Study the drawing (mm; zero at the part's minimum x, y, z) and answer. A direction names the side the tool comes from. Coordinates: 2 decimals unless noted, no trailing zeros. Write each loop counter-clockwise with the first axis right and the second up, starting at its lowest first coordinate (ties: lowest second). Pieces come first, ordered by that corner, then holes. Notation, with made-up numbers: (-23, 43) -> (17, 43) arc R20 cw to (17, 72) -> close; hole circle Ø1 at (10.25, 11). An arc over 180 degrees is marked (long way). Answer in a Markdown table with one row per item. Add a question column.
Item 1: Section B-B on x = 110.5 is taken. Write down the section's boundary in (y, z).
Item 2: Given pin 1 Ø12 at (x, y) = (30, 64.5) entering from -Z; pin 2 Ø3 at (x, y) = (14, 101.5) entering from +Z, each flat-ended and moving along its own axis, determine where each tip first touches the part or whether it passes through.
Item 3: Which of the six approach directions +Z, -Z, +X, -X, +Y, -Y give full straight-line access (tool end or side, diameter ignored) to the marked faces 1, 2 and 3?
Item 4: Straight lines are drawn through the part: line 1 (Z direction, x = 122.5, y = 21); line 2 (Y direction, x = 22.5, z = 41.5); line 3 (Y direction, x = 21.5, z = 71.5). For each, find the intervals that lie inside material, in ascending order. Write a range as from..to.
Item 5: Section A-A on y = 35.5 is taken. Write down the section's boundary in (x, z).
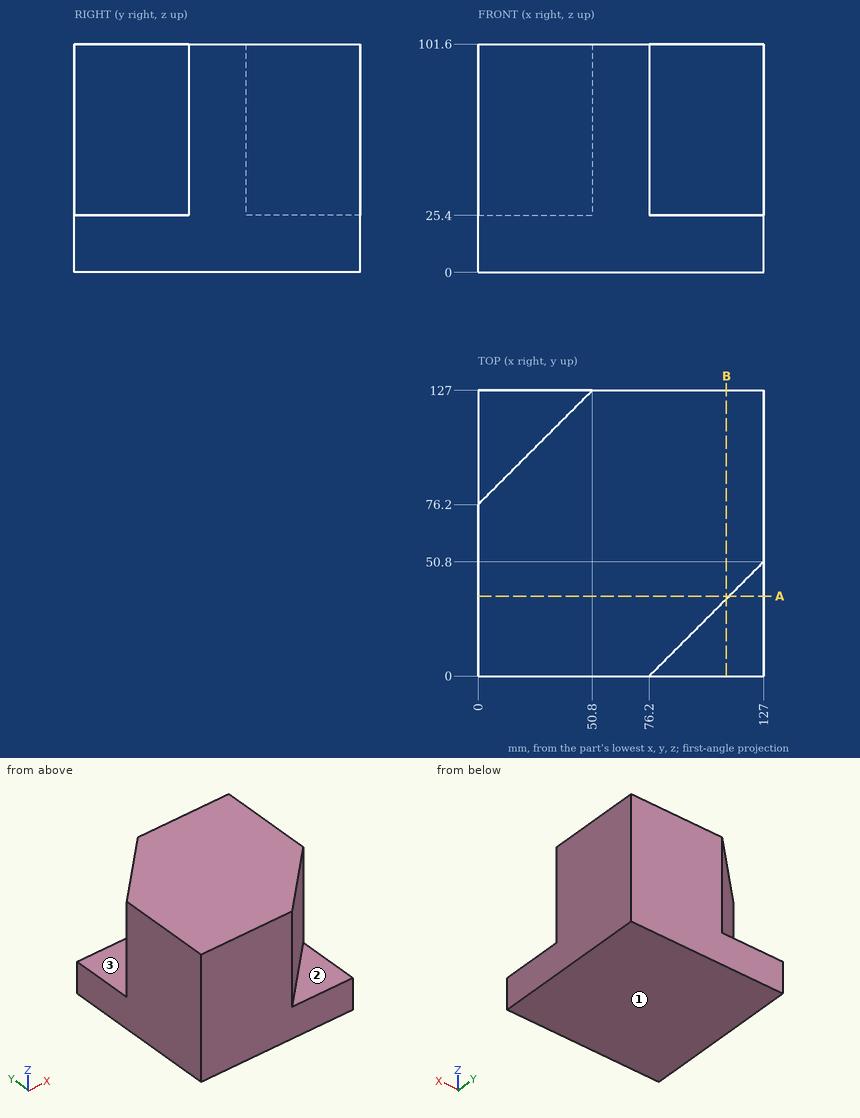
Results below:
| question | item | result |
|---|---|---|
| 1 | outline | (0, 0) -> (127, 0) -> (127, 101.6) -> (34.3, 101.6) -> (34.3, 25.4) -> (0, 25.4) -> close |
| 2 | pin 1 | stops at z = 0 |
| 2 | pin 2 | stops at z = 25.4 |
| 3 | face 1 | -Z, +X, -X, +Y, -Y |
| 3 | face 2 | +Z, +X, -Y |
| 3 | face 3 | +Z, -X, +Y |
| 4 | line 1 | z = 0..25.4 |
| 4 | line 2 | y = 0..98.7 |
| 4 | line 3 | y = 0..97.7 |
| 5 | outline | (0, 0) -> (127, 0) -> (127, 25.4) -> (111.7, 25.4) -> (111.7, 101.6) -> (0, 101.6) -> close |
